Design review of the part built by this model. Coordinates are the model's own, in mm. A direction names the side the tool comes from. Give positions to 0.01 mm unless a question says otherwise; leave off trailing zeros. Order: outer loops, then holes, each group sorted by start corner. A loop starts at its lowest first (then second) coordinate and runs counter-clockwise, first axis right, second up. Notation, with made-up numbers: (-7, 75) -> (13, 75) arc R18 ccw to (13, 79) -> close; hole circle Ø6 at (19, -23.75). An arc over 180 degrees is marked (long way). Return JSON: item names as keys, results as strings.
```python
from build123d import *

# Parameters (mm, degrees)
SKETCH1_R           = 11.1125
SKETCH1_R_2         = 4.7625
BOSS_EXTRUDE1_DEPTH = 23.495
SKETCH2_R           = 4.7625
BOSS_EXTRUDE2_DEPTH = 6.35
SKETCH3_W           = 31.75
SKETCH3_H           = 3.175
BOSS_EXTRUDE3_DEPTH = 25.4
BOSS_EXTRUDE4_DEPTH = 3.175
BOSS_EXTRUDE5_DEPTH = 3.175
SKETCH6_R           = 1.5
CUT_EXTRUDE1_DEPTH  = 12.319
FILLET1_R           = 1.5875


with BuildPart() as part:
    # Sketch1 → Boss-Extrude1 (new body)
    with BuildSketch(Plane.XY):
        Circle(SKETCH1_R)
        Circle(SKETCH1_R_2, mode=Mode.SUBTRACT)
    extrude(amount=BOSS_EXTRUDE1_DEPTH)

    # Sketch2 → Boss-Extrude2 (add)
    with BuildSketch(Plane(origin=(0, 0, 0), x_dir=(-1, 0, 0), z_dir=(0, 0, -1))):
        with BuildLine():
            Line((15.875, -28.575), (15.875, 0))
            ThreePointArc((15.875, 0), (0, 15.875), (-15.875, 0))
            Line((-15.875, 0), (-15.875, -28.575))
            Line((-15.875, -28.575), (15.875, -28.575))
        make_face()
        Circle(SKETCH2_R, mode=Mode.SUBTRACT)
    extrude(amount=BOSS_EXTRUDE2_DEPTH)

    # Sketch3 → Boss-Extrude3 (add)
    with BuildSketch(Plane(origin=(0, 0, -6.35), x_dir=(-1, 0, 0), z_dir=(0, 0, -1))):
        with Locations((0, -26.9875)):
            Rectangle(SKETCH3_W, SKETCH3_H)
    extrude(amount=BOSS_EXTRUDE3_DEPTH)

    # Sketch4 → Boss-Extrude4 (add)
    with BuildSketch(Plane.ZY.offset(15.875)):
        Polygon((-31.75, -25.4), (-6.35, 0), (-6.35, -25.4), align=None)
    extrude(amount=-BOSS_EXTRUDE4_DEPTH)

    # Sketch5 → Boss-Extrude5 (add)
    with BuildSketch(Plane(origin=(15.875, 0, 0), x_dir=(0, 0, -1), z_dir=(1, 0, 0))):
        Polygon((6.35, -25.4), (31.75, -25.4), (6.35, 0), align=None)
    extrude(amount=-BOSS_EXTRUDE5_DEPTH)

    # Sketch6 → Cut-Extrude1 (cut)
    with BuildSketch(Plane(origin=(0, -25.4, 0), x_dir=(1, 0, 0), z_dir=(0, 1, 0))):
        with Locations((-9.525, 28.575)):
            Circle(SKETCH6_R)
        with Locations((9.525, 28.575)):
            Circle(SKETCH6_R)
        with Locations((9.525, 9.525)):
            Circle(SKETCH6_R)
        with Locations((-9.525, 9.525)):
            Circle(SKETCH6_R)
    extrude(amount=-CUT_EXTRUDE1_DEPTH, mode=Mode.SUBTRACT)

    # Fillet1
    fillet1_edges = [part.edges().sort_by_distance(p)[0] for p in [
        (-11.1125, 0, 23.495),
    ]]
    fillet(fillet1_edges, radius=FILLET1_R)


solid = part.part
```
Item 1: For pin 1 (3.5 mm diameter, centred on x = -9.525, z = -9.525, fed in from +Y); pin 2 (9.5 mm diameter, centred on x = -5, y = -10.5, fed in from -Z); pin 3 (6 mm diameter, centred on x = -4, y = -12.5, fed in from +Z); pin 4 (7.5 mm diameter, centred on x = 0, y = 0, fed in from -Z), all flat-tipped, find the tip position at first contact; note any pin that passes through.
Result set:
{"pin 1": "stops at y = -25.4", "pin 2": "stops at z = -6.35", "pin 3": "stops at z = 23.38", "pin 4": "passes through"}
Item 2: Wall thickness on L1, parallel to X at y = -23.5, z = -14.5 (3 decimals); L2, parallel to Y at x = 0, z = 13; L3, parallel to Y at x = 0, z = -4 (1 decimal): over which ranges is each line inside the solid? List them lowest first. Write a range as [from, to].
Result set:
{"L1": "x = [-15.875, -12.7], [12.7, 15.875]", "L2": "y = [-11.11, -4.76], [4.76, 11.11]", "L3": "y = [-28.6, -4.8], [4.8, 15.9]"}
Item 3: Add section C-C (y = -19). Give the boundary of the cut face in (x, z) (3 decimals).
Result set:
{"outline": "(-15.875, -25.35) -> (-12.7, -25.35) -> (-12.7, -6.35) -> (12.7, -6.35) -> (12.7, -25.35) -> (15.875, -25.35) -> (15.875, 0) -> (-15.875, 0) -> close"}
Item 4: Mouldability with a two-part tool opening along X and no side actions: class faces 1 (the face through (15.875, -17, -12)), 2 (the face through (-12.7, -18, -13)), 3 (the face through (14.31, -12.88, -19.23)) as released by +X, released by -X, zero draft, split by the parting line, or undercut.
Result set:
{"face 1": "released by +X", "face 2": "undercut", "face 3": "zero draft"}
Item 5: Machinability: for faces 4 (the face through (12.7, -18, -13)), 5 (the face through (10.6, 3.34, 10.8)), 6 (the face through (-8.833, -26.965, -27.244)), which of the approach directions +Z, -Z, +X, -X, +Y, -Y give a long, thin tool a straight path to every point of the face, cutting with its end or side? Answer none if there is none.
Result set:
{"face 4": "-Z, +Y", "face 5": "+Z", "face 6": "+Y, -Y"}
Item 6: Add section D-D (z = 15). Give the boundary of the cut face in (x, y) (1 decimal), plus the area to 3 significant figures.
Result set:
{"outline": "circle Ø22.2 at (0, 0); hole circle Ø9.5 at (0, 0)", "area": "317 mm^2"}
Item 7: Add section B-B (z = -12.5). Give the boundary of the cut face in (x, y) (3 decimals), plus the area to 3 significant figures.
Result set:
{"outline": "(-15.875, -28.575) -> (15.875, -28.575) -> (15.875, -6.15) -> (12.7, -6.15) -> (12.7, -25.4) -> (-12.7, -25.4) -> (-12.7, -6.15) -> (-15.875, -6.15) -> close", "area": "223 mm^2"}
